The listing builds one solid part. Answer for the finished solid, in the listing's coordinates (mm). Face numbers are marked on the shaded views. A direction names the side the tool comes from. Round coordinates to 2 decimals unless told otherwise and drop trailing zeros. Order: outer loops, then holes, each group sorted by start corner. A loop starts at its lowest first (then second) coordinate and runs counter-clockwise, first axis right, second up. Notation, with made-up numbers: M 21.5,54.25 L 29.5,54.25 A23 ccw 29.5,81.25 Z; hole C 49.5,12.25 d2. An arc over 180 degrees is marked long. Write item = value, one per line. Start each with the question number.
(1) A cutting plane is placed at C-C, the plane z = 18.5. Determine the outline of the cut face in (x, y), and give its area (3 significant figures).
(2) Which of the six approach directions +Z, -Z, +X, -X, +Y, -Y give full straight-line access (tool end or side, diameter ignored) to the marked faces 1 and 2?
(3) A cutting plane is placed at A-A, the plane x = 0. Determine the outline of the cut face in (y, z) (3 decimals), and give its area (3 significant figures).
(4) Each of these flat-tipped pins is pushed along its axis until it touches: pin 1 (3 mm diameter, centred on x = -3, z = 105.5, fed in from +Y); pin 2 (2 mm diameter, centred on x = -4, z = 138, fed in from -Y); pin 3 (3 mm diameter, centred on x = -5.5, z = 99.5, fed in from -Y). Where does it stop, or does it pass through?
(5) Straight lines are drawn through the part: probe 1 along Y at (x, z) = (0, -5) (3 decimals); probe 2 along Z at (x, y) = (3.75, -4.5); probe 3 along Z at (x, y) = (5.25, 3.25). For each, find the intervals that lie inside material, in ascending order. Write a range as from..to.
(6) A cutting plane is placed at D-D, the plane z = 143.5. Determine the outline of the cut face in (x, y) (3 decimals).
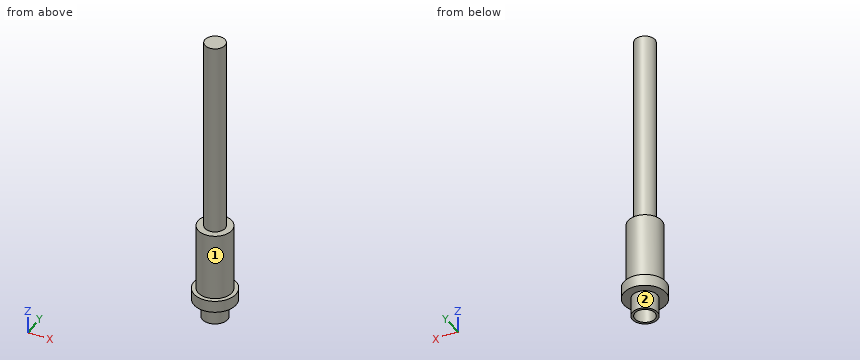
from build123d import *

# Parameters (mm, degrees)
F0_R      = 7.485
F0_R_2    = 5.985
F1_DEPTH  = 11
F2_R      = 7.485
F2_R_2    = 5.985
F3_DEPTH  = 7
F2_R_3    = 12.5
F4_DEPTH  = 7
F5_R      = 10
F6_DEPTH  = 40.05
F9_R      = 5.985
F10_DEPTH = 117.5055425


# Not quite as in the source:
# - an extrude ends at something that could not be found from the text; its depth is read off the source's solid
# - the program builds the solid bodies; features that only make, move or delete a surface that nothing else refers to are left out


with BuildPart() as f1:
    # F0 (on Top) → F1 (new body)
    with BuildSketch(Plane.XY):
        Circle(F0_R)
        Circle(F0_R_2, mode=Mode.SUBTRACT)
    extrude(amount=-F1_DEPTH)

    # F2 (on face) → F3 (join)
    with BuildSketch(Plane.XY):
        Circle(F2_R)
        Circle(F2_R_2, mode=Mode.SUBTRACT)
    extrude(amount=F3_DEPTH)

    # F2 (on face) → F4 (join)
    with BuildSketch(Plane.XY):
        Circle(F2_R_3)
    extrude(amount=F4_DEPTH)

    # F5 (on face) → F6 (join)
    with BuildSketch(Plane.XY.offset(7)):
        Circle(F5_R)
    extrude(amount=F6_DEPTH)

    # F9 (on face) → F10 (join, through all)
    with BuildSketch(Plane.XY.offset(47.05)):
        Circle(F9_R)
    extrude(amount=F10_DEPTH)


solid = f1.part
Reported:
q1.outline = C 0,0 d20
q1.area = 314 mm²
q2.face_1 = +Z
q2.face_2 = -Z
q3.outline = M -12.5,0 L -7.485,0 L -7.485,-11 L -5.985,-11 L -5.985,0 L 5.985,0 L 5.985,-11 L 7.485,-11 L 7.485,0 L 12.5,0 L 12.5,7 L 10,7 L 10,47.05 L 5.985,47.05 L 5.985,164.556 L -5.985,164.556 L -5.985,47.05 L -10,47.05 L -10,7 L -12.5,7 Z
q3.area = 2,420 mm²
q4.pin_1 = 5.79
q4.pin_2 = -5.18
q4.pin_3 = -4.45
q5.probe_1 = -7.485..-5.985, 5.985..7.485
q5.probe_2 = 0..164.56
q5.probe_3 = -11..47.05
q6.outline = C 0,0 d11.97
